from build123d import *

# Parameters (mm, degrees)
F0_W     = 2.5
F0_H     = 20
F0_W_2   = 4
F0_W_3   = 8.5
F1_DEPTH = 2.5
F2_DEPTH = 12
F3_DEPTH = 12
F4_DEPTH = 36
F5_START = 33.6
F5_DEPTH = 2.4
F6_R     = 2
F7_START = 32.6
F7_DEPTH = 3.4
F8_SIZE  = 0.5


with BuildPart() as f1:
    # F0 (on Top) → F1 (new body)
    with BuildSketch(Plane.XY):
        with BuildLine():
            ThreePointArc((-40.6337848902, 13.9120002314), (-41.3863019049, 16.2473490834), (-40.6337848902, 18.5826979354))
            Line((-40.6337848902, 18.5826979354), (-40.6337848902, 26.2473490834))
            Line((-40.6337848902, 26.2473490834), (-43.1337848902, 26.2473490834))
            Line((-43.1337848902, 26.2473490834), (-43.1337848902, 6.2473490834))
            Line((-43.1337848902, 6.2473490834), (-40.6337848902, 6.2473490834))
            Line((-40.6337848902, 6.2473490834), (-40.6337848902, 13.9120002314))
        make_face()
        with BuildLine():
            ThreePointArc((-40.6337848902, 18.5826979354), (-36.159503621, 20.0545745785), (-33.3863019049, 16.2473490834))
            ThreePointArc((-33.3863019049, 16.2473490834), (-36.159503621, 12.4401235883), (-40.6337848902, 13.9120002314))
            Line((-40.6337848902, 13.9120002314), (-40.6337848902, 6.2473490834))
            Line((-40.6337848902, 6.2473490834), (-20.8337848902, 6.2473490834))
            Line((-20.8337848902, 6.2473490834), (-20.8337848902, 26.2473490834))
            Line((-20.8337848902, 26.2473490834), (-40.6337848902, 26.2473490834))
            Line((-40.6337848902, 26.2473490834), (-40.6337848902, 18.5826979354))
        make_face()
        with BuildLine():
            Line((-40.6337848902, 13.9120002314), (-40.6337848902, 18.5826979354))
            ThreePointArc((-40.6337848902, 18.5826979354), (-41.3863019049, 16.2473490834), (-40.6337848902, 13.9120002314))
        make_face()
        with BuildLine():
            ThreePointArc((-40.6337848902, 13.9120002314), (-36.159503621, 12.4401235883), (-33.3863019049, 16.2473490834))
            ThreePointArc((-33.3863019049, 16.2473490834), (-36.159503621, 20.0545745785), (-40.6337848902, 18.5826979354))
            Line((-40.6337848902, 18.5826979354), (-40.6337848902, 13.9120002314))
        make_face()
        with Locations((-19.5837848902, 16.2473490834)):
            Rectangle(F0_W, F0_H)
        with Locations((-53.6337848902, 16.2473490834)):
            Rectangle(F0_W_2, F0_H)
        with Locations((-47.3837848902, 16.2473490834)):
            Rectangle(F0_W_3, F0_H)
    extrude(amount=F1_DEPTH)

    # F0 (on Top) → F2 (join)
    with BuildSketch(Plane.XY):
        with Locations((-19.5837848902, 16.2473490834)):
            Rectangle(F0_W, F0_H)
    extrude(amount=F2_DEPTH)

    # F0 (on Top) → F3 (join)
    with BuildSketch(Plane.XY):
        with BuildLine():
            Line((-40.6337848902, 13.9120002314), (-40.6337848902, 18.5826979354))
            ThreePointArc((-40.6337848902, 18.5826979354), (-41.3863019049, 16.2473490834), (-40.6337848902, 13.9120002314))
        make_face()
        with BuildLine():
            ThreePointArc((-40.6337848902, 13.9120002314), (-36.159503621, 12.4401235883), (-33.3863019049, 16.2473490834))
            ThreePointArc((-33.3863019049, 16.2473490834), (-36.159503621, 20.0545745785), (-40.6337848902, 18.5826979354))
            Line((-40.6337848902, 18.5826979354), (-40.6337848902, 13.9120002314))
        make_face()
    extrude(amount=F3_DEPTH)

    # F0 (on Top) → F4 (join)
    with BuildSketch(Plane.XY):
        with Locations((-53.6337848902, 16.2473490834)):
            Rectangle(F0_W_2, F0_H)
    extrude(amount=F4_DEPTH)

    # F0 (on Top) → F5 (join)
    with BuildSketch(Plane.XY.offset(F5_START)):
        with Locations((-47.3837848902, 16.2473490834)):
            Rectangle(F0_W_3, F0_H)
    extrude(amount=F5_DEPTH)

    # F6
    f6_edges = [f1.edges().sort_by_distance(p)[0] for p in [
        (-34.138819, 18.582698, 12),
    ]]
    fillet(f6_edges, radius=F6_R)

    # F0 (on Top) → F7 (join)
    with BuildSketch(Plane.XY.offset(F7_START)):
        with BuildLine():
            ThreePointArc((-40.6337848902, 13.9120002314), (-41.3863019049, 16.2473490834), (-40.6337848902, 18.5826979354))
            Line((-40.6337848902, 18.5826979354), (-40.6337848902, 26.2473490834))
            Line((-40.6337848902, 26.2473490834), (-43.1337848902, 26.2473490834))
            Line((-43.1337848902, 26.2473490834), (-43.1337848902, 6.2473490834))
            Line((-43.1337848902, 6.2473490834), (-40.6337848902, 6.2473490834))
            Line((-40.6337848902, 6.2473490834), (-40.6337848902, 13.9120002314))
        make_face()
        with BuildLine():
            Line((-40.6337848902, 13.9120002314), (-40.6337848902, 18.5826979354))
            ThreePointArc((-40.6337848902, 18.5826979354), (-41.3863019049, 16.2473490834), (-40.6337848902, 13.9120002314))
        make_face()
    extrude(amount=F7_DEPTH)

    # F8
    f8_edges = [f1.edges().sort_by_distance(p)[0] for p in [
        (-40.633785, 16.247349, 32.6),
        (-43.133785, 16.247349, 32.6),
    ]]
    chamfer(f8_edges, length=F8_SIZE)


solid = f1.part
Could you check a few things on this model? Use its own coordinates, in mm. A direction names the side the tool comes from. Round coordinates to 2 decimals unless told otherwise and drop trailing zeros. Order: outer loops, then holes, each group sorted by start corner. A loop starts at its lowest first (then second) coordinate and runs counter-clockwise, first axis right, second up.
(1) Imagine slicing it at C-C (z = 23). Write out the boundary of the cut face in (x, y).
Response values:
outline: (-55.63, 6.25) - (-51.63, 6.25) - (-51.63, 26.25) - (-55.63, 26.25) - close
(2) Imagine slicing it at D-D (x = -28). Write out the boundary of the cut face in (y, z).
Response values:
outline: (6.25, 0) - (26.25, 0) - (26.25, 2.5) - (6.25, 2.5) - close
(3) Please list where these lines run through material, in increasing order: line 1 along Z through (x, y) = (-44, 16); line 2 along Z through (x, y) = (-42, 13.75); line 3 along Z through (x, y) = (-23.5, 11.5).
Response values:
line 1: z = 0 to 2.5, 33.6 to 36
line 2: z = 0 to 2.5, 32.6 to 36
line 3: z = 0 to 2.5
(4) If we mould it in two halves opening along Z, with no side actions, what happens to faces 1 (the flat face through (-51.634, 16, 18)), 2 (the flat face through (-42, 16, 32.6)), 3 (the flat face through (-20, 16, 12)), 4 (the flat face through (-55.634, 16, 18))? For each: released by +Z, released by -Z, zero draft, split by the parting line, or undercut.
Response values:
face 1: undercut
face 2: undercut
face 3: released by +Z
face 4: zero draft
(5) Which directions (+Z, -Z, +X, -X, +Y, -Y) give clear straight access to the entire face, cutting with the end or side of a thin tool? Please do faces 5 (the flat face through (-18.334, 16, 6)), 6 (the flat face through (-20.834, 16, 7)), 7 (the flat face through (-52, 6.247, 13)), 8 (the flat face through (-40.634, 16, 35)), 9 (the flat face through (-47, 16, 33.6)).
Response values:
face 5: +Z, -Z, +X, +Y, -Y
face 6: +Z, +Y, -Y
face 7: +Z, -Z, +X, -X, -Y
face 8: +Z, +X, +Y, -Y
face 9: +Y, -Y
(6) Imagine slicing it at B-B (y = 10). Write out the boundary of the cut face in (x, z), plus the area to 3 significant figures.
Response values:
outline: (-55.63, 0) - (-18.33, 0) - (-18.33, 12) - (-20.83, 12) - (-20.83, 2.5) - (-51.63, 2.5) - (-51.63, 33.6) - (-43.13, 33.6) - (-43.13, 33.1) - (-42.63, 32.6) - (-41.13, 32.6) - (-40.63, 33.1) - (-40.63, 36) - (-55.63, 36) - close
area: 280 mm2
(7) Imagine slicing it at A-A (x = -46). Write out the boundary of the cut face in (y, z).
Response values:
outline: (6.25, 0) - (26.25, 0) - (26.25, 2.5) - (6.25, 2.5) - close; (6.25, 33.6) - (26.25, 33.6) - (26.25, 36) - (6.25, 36) - close
(8) I'm going to push flat-ended pins straight in: pin 1 (4 mm diameter, centred on x = -26.5, y = 23.5, fed in from +Z); pin 2 (0.9 mm diameter, centred on y = 16.5, z = 35, fed in from +X); pin 3 (3 mm diameter, centred on x = -19, y = 13.5, fed in from +Z). Where does each tip first touch, or does it pass through?
Response values:
pin 1: stops at z = 2.5
pin 2: stops at x = -40.63
pin 3: stops at z = 12
